Model file for the job. Use its own axes, mm. Face numbers are marked on the shaded views. A direction names the side the tool comes from. Coordinates: 2 decimals unless noted, no trailing zeros. Write each loop counter-clockwise with the first axis right and the second up, starting at its lowest first coordinate (ties: lowest second). Pieces come first, ordered by that corner, then holes. Notation, with made-up numbers: (-21, 8) - (17, 8) arc R13 ccw to (17, 28) - close; hole circle Ø5 at (-3.75, -9.5). An arc over 180 degrees is marked (long way). Put each result on its own line as item: value. Start each with the question number.
1. Saw through at A-A, the plane y = -2.75. Write the cut outline in (x, z), plus the area to 3 significant figures.
2. Drop flat-ended pins along their axis: P1, Ø1.8, axis at y = -1.5, z = 18, coming from the +X side; P2, Ø2, axis at y = -1.5, z = 18.5, coming from the -X side. Give the stop position or say it passes through.
3. Drill centre lines: L1, parallel to Z at x = 23, y = -0.5; L2, parallel to Z at x = 39, y = -1; L3, parallel to X at y = -0.25, z = 16.75. Where is each one in solid material? Low to high. Write a range as from..to.
4. Saw through at B-B, the plane x = 22.5. Write the cut outline in (y, z), plus the area to 3 significant figures.
5. Which spindle directions (+Z, -Z, +X, -X, +Y, -Y) get a long thin tool onto all of the face, cutting with end or side? Do the marked faces 1, 2, 3, 4 and 5. Say none if no direction does.
6. Saw through at D-D, the plane z = 17.25. Write the cut outline in (x, y).
7. Pull direction Z, two halves, no side cores. Call the marked faces 6, 7 and 8: released by +Z, released by -Z, zero draft, split by the parting line, or undercut.
8. Saw through at C-C, the plane y = 1.75. Write the cut outline in (x, z), plus the area to 3 significant figures.
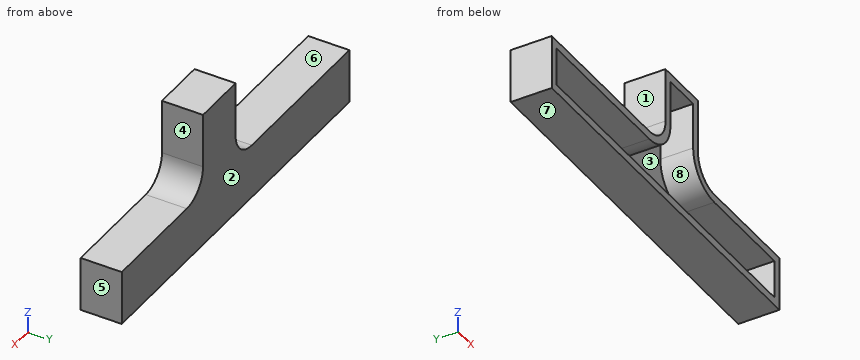
```python
from build123d import *

# Parameters (mm, degrees)
F2_DEPTH = 5
F3_DEPTH = 2.5
F4_T     = -1.5


with BuildPart() as f2:
    # F0 (on Front) → F2 (new body)
    with BuildSketch(Plane.XZ):
        with BuildLine():
            Line((0, 10), (0, 0))
            Line((0, 0), (70, 0))
            Line((70, 0), (70, 10))
            Line((70, 10), (50, 10))
            ThreePointArc((50, 10), (46.464466, 11.464466), (45, 15))
            Line((45, 15), (45, 25))
            Line((45, 25), (35, 25))
            Line((35, 25), (35, 15))
            ThreePointArc((35, 15), (33.535534, 11.464466), (30, 10))
            Line((30, 10), (0, 10))
        make_face()
    extrude(amount=F2_DEPTH)

    # F0 (on Front) → F3 (join, symmetric)
    with BuildSketch(Plane.XZ):
        with BuildLine():
            Line((0, 10), (0, 0))
            Line((0, 0), (70, 0))
            Line((70, 0), (70, 10))
            Line((70, 10), (50, 10))
            ThreePointArc((50, 10), (46.464466, 11.464466), (45, 15))
            Line((45, 15), (45, 25))
            Line((45, 25), (35, 25))
            Line((35, 25), (35, 15))
            ThreePointArc((35, 15), (33.535534, 11.464466), (30, 10))
            Line((30, 10), (0, 10))
        make_face()
    extrude(amount=F3_DEPTH, both=True)

    # F4
    f4_openings = [f2.faces().sort_by_distance(p)[0] for p in [
        (35.933685, -5, 7.254637),
    ]]
    offset(amount=F4_T, openings=f4_openings)


solid = f2.part
```
Final values:
1. outline: (0, 0) - (70, 0) - (70, 10) - (50, 10) arc R5 cw to (45, 15) - (45, 25) - (35, 25) - (35, 15) arc R5 cw to (30, 10) - (0, 10) - close; hole (1.5, 1.5) - (68.5, 1.5) - (68.5, 8.5) - (50, 8.5) arc R6.5 cw to (43.5, 15) - (43.5, 23.5) - (36.5, 23.5) - (36.5, 15) arc R6.5 cw to (30, 8.5) - (1.5, 8.5) - close
1. area: 269 mm²
2. P1: stops at x = 45
2. P2: stops at x = 35
3. L1: z = 0..1.5, 8.5..10
3. L2: z = 0..1.5, 23.5..25
3. L3: x = 35..36.5, 43.5..45
4. outline: (-5, 0) - (2.5, 0) - (2.5, 10) - (-5, 10) - (-5, 8.5) - (1, 8.5) - (1, 1.5) - (-5, 1.5) - close
4. area: 33.0 mm²
5. face 1: +Z, -X, +Y, -Y
5. face 2: +Z, -Z, +X, -X, +Y
5. face 3: -Y
5. face 4: +Z, +X, +Y, -Y
5. face 5: +Z, -Z, +X, +Y, -Y
6. outline: (35, -5) - (36.5, -5) - (36.5, 1) - (43.5, 1) - (43.5, -5) - (45, -5) - (45, 2.5) - (35, 2.5) - close
7. face 6: released by +Z
7. face 7: released by -Z
7. face 8: undercut
8. outline: (0, 0) - (70, 0) - (70, 10) - (50, 10) arc R5 cw to (45, 15) - (45, 25) - (35, 25) - (35, 15) arc R5 cw to (30, 10) - (0, 10) - close
8. area: 861 mm²
